Read the model definition and answer for the solid it produces. Units are mm, in the model's axes. Give positions to 0.01 mm unless a question says otherwise; leave off trailing zeros. Order: outer loops, then holes, each group sorted by start corner. A loop starts at its lowest first (then second) coordinate and runs counter-clockwise, first axis right, second up. Notation, with made-up numbers: (-37.5, 41.5) -> (-24.5, 41.5) arc R32 ccw to (-24.5, 75.5) -> close; hole circle Ø9 at (65, 58). An arc over 180 degrees is marked (long way). Answer as CSV lines item,"result". Start each with the question number.
1) Find section A-A (x = 2.1). State how many separate pieces and enclosed holes the cut face has, and give its area (3 significant figures).
2) Straight lines are drawn through the part: L1, parallel to Y at x = 1.5, z = 0; L2, parallel to Z at x = 0.45, y = 23; L3, parallel to Z at x = 1.7, y = -2. For each, find the intervals that lie inside material, in ascending order. Write a range as from..to.
3) Find section B-B (y = 60). Determine the outline of the cut face in (x, z), and give its area (3 significant figures).
4) The mould has two halves that part along Y. Classify faces 1 (the face through (1.52, 23.26, -37.43)), 2 (the face through (1, 70, 1)), 3 (the face through (0, 38, -1)): +Y half, -Y half, draft (parallel to the pull), parting line (faces both ways), or undercut.
5) Flat-ended cylindrical pins translate along their axes: pin 1 Ø1 at (y, z) = (23.5, 37.5) entering from -X; pin 2 Ø1 at (x, y) = (0.5, -12) entering from +Z. Find the tip coordinate at first contact, or state that the pin passes through.
6) Find section C-C (z = -28.5). Determine the outline of the cut face in (x, y), and give its area (3 significant figures).
7) Find section D-D (y = -34). Determine the outline of the cut face in (x, z).
```python
from build123d import *

# Parameters (mm, degrees)
SKETCH_1_R          = 50
SKETCH_1_R_2        = 36
EXTRUDE_1_DEPTH     = 3
EXTRUDE_START       = -3
EXTRUDE_2_DEPTH     = 3
SKETCH_3_R          = 1.5
CUT_EXTRUDE_1_DEPTH = 3
SKETCH_4_R          = 2.1
CUT_EXTRUDE_2_DEPTH = 87.075548212
FILLET_2_R          = 5


with BuildPart() as part:
    # 草图1 → 凸台-拉伸1 (new body)
    with BuildSketch(Plane(origin=(0, 0, 0), x_dir=(0, 0, -1), z_dir=(1, 0, 0))):
        Circle(SKETCH_1_R)
        Circle(SKETCH_1_R_2, mode=Mode.SUBTRACT)
    extrude(amount=EXTRUDE_1_DEPTH)

    # 草图2 → 凸台-拉伸2 (add)
    with BuildSketch(Plane(origin=(3, 0, 0), x_dir=(0, 0, -1), z_dir=(1, 0, 0)).offset(EXTRUDE_START)):
        with BuildLine():
            Line((-50, 0), (-50, 70))
            Line((-50, 70), (50, 70))
            Line((50, 70), (50, 0))
            ThreePointArc((50, 0), (0, 50), (-50, 0))
        make_face()
    extrude(amount=EXTRUDE_2_DEPTH)

    # 草图3 → 切除-拉伸1 (cut)
    with BuildSketch(Plane(origin=(3, 0, 0), x_dir=(0, 0, -1), z_dir=(1, 0, 0))):
        with Locations((0, 44.5)):
            Circle(SKETCH_3_R)
        with Locations((38.538130468, 22.25)):
            Circle(SKETCH_3_R)
        with Locations((38.538130468, -22.25)):
            Circle(SKETCH_3_R)
        with Locations((0, -44.5)):
            Circle(SKETCH_3_R)
        with Locations((-38.538130468, -22.25)):
            Circle(SKETCH_3_R)
        with Locations((-38.538130468, 22.25)):
            Circle(SKETCH_3_R)
    extrude(amount=-CUT_EXTRUDE_1_DEPTH, mode=Mode.SUBTRACT)

    # 草图4 → 切除-拉伸2 (cut, through all)
    with BuildSketch(Plane(origin=(3, 0, 0), x_dir=(0, 0, -1), z_dir=(1, 0, 0))):
        with Locations((-40, 60)):
            Circle(SKETCH_4_R)
        with Locations((0, 60)):
            Circle(SKETCH_4_R)
        with Locations((40, 60)):
            Circle(SKETCH_4_R)
    extrude(amount=-CUT_EXTRUDE_2_DEPTH, mode=Mode.SUBTRACT)

    # 圆角2
    fillet_2_edges = [part.edges().sort_by_distance(p)[0] for p in [
        (1.5, 70, 50),
        (1.5, 70, -50),
    ]]
    fillet(fillet_2_edges, radius=FILLET_2_R)


solid = part.part
```
Findings below:
1,separate pieces,"1"
1,enclosed holes,"10"
1,area,"6,760 mm²"
2,L1,"-50..-46, -43..-36, 36..43, 46..57.9, 62.1..70"
2,L2,"-50..-39.84, -37.24..-27.69, 27.69..37.24, 39.84..50"
2,L3,"-49.96..-35.94, 35.94..49.96"
3,outline,"(0, -50) -> (3, -50) -> (3, -42.1) -> (0, -42.1) -> close; (0, -37.9) -> (3, -37.9) -> (3, -2.1) -> (0, -2.1) -> close; (0, 2.1) -> (3, 2.1) -> (3, 37.9) -> (0, 37.9) -> close; (0, 42.1) -> (3, 42.1) -> (3, 50) -> (0, 50) -> close"
3,area,"262 mm²"
4,face 1,"undercut"
4,face 2,"+Y half"
4,face 3,"draft"
5,pin 1,"x = 0"
5,pin 2,"z = 48.66"
6,outline,"(0, -41.08) -> (3, -41.08) -> (3, -21.99) -> (0, -21.99) -> close; (0, 21.99) -> (3, 21.99) -> (3, 70) -> (0, 70) -> close"
6,area,"201 mm²"
7,outline,"(0, -36.66) -> (3, -36.66) -> (3, -11.83) -> (0, -11.83) -> close; (0, 11.83) -> (3, 11.83) -> (3, 36.66) -> (0, 36.66) -> close"
